Here's how the part is built. I have some questions about the finished solid (model axes, mm). A direction names the side the tool comes from. Round coordinates to 2 decimals unless told otherwise and drop trailing zeros. Write each loop counter-clockwise with the first axis right and the second up, starting at its lowest first coordinate (ties: lowest second). Pieces come first, ordered by that corner, then holes. Notation, with made-up numbers: (48, -1.5) -> (105, -1.5) arc R8 cw to (105, 7.5) -> close; hole circle Ø7 at (-5, -38.5). An arc over 180 degrees is marked (long way). Answer as CSV lines item,"result".
from build123d import *

# Parameters (mm, degrees)
SKETCH1_R           = 11
BOSS_EXTRUDE2_DEPTH = 13
SKETCH4_W           = 38
SKETCH4_H           = 51
BOSS_EXTRUDE3_DEPTH = 45
CUT_EXTRUDE1_DEPTH  = 45
BOSS_EXTRUDE4_DEPTH = 45
SKETCH15_R          = 11
BOSS_EXTRUDE6_DEPTH = 10
SKETCH16_R          = 11
BOSS_EXTRUDE7_DEPTH = 10


with BuildPart() as part:
    # Sketch1 → Boss-Extrude2 (new body)
    with BuildSketch(Plane(origin=(0, 0, 0), x_dir=(1, 0, 0), z_dir=(0, 1, 0))):
        with BuildLine():
            Line((-57, 32), (57, 32))
            ThreePointArc((57, 32), (89, 0), (57, -32))
            Line((57, -32), (-57, -32))
            ThreePointArc((-57, -32), (-89, 0), (-57, 32))
        make_face()
        with Locations(Location((-57, 0, 0), (0, 0, 90))):
            Circle(SKETCH1_R, mode=Mode.SUBTRACT)
        with Locations(Location((57, 0, 0), (0, 0, 90))):
            Circle(SKETCH1_R, mode=Mode.SUBTRACT)
    extrude(amount=BOSS_EXTRUDE2_DEPTH)

    # Sketch4 → Boss-Extrude3 (add)
    with BuildSketch(Plane(origin=(0, 13, 0), x_dir=(1, 0, 0), z_dir=(0, 1, 0))):
        with Locations((0, -6.5)):
            Rectangle(SKETCH4_W, SKETCH4_H)
    extrude(amount=BOSS_EXTRUDE3_DEPTH)

    # Sketch5 → Cut-Extrude1 (cut)
    with BuildSketch(Plane(origin=(19, 0, 0), x_dir=(0, 0, -1), z_dir=(1, 0, 0))):
        Polygon((19, 58), (-32, 13), (-32, 58), align=None)
    extrude(amount=-CUT_EXTRUDE1_DEPTH, mode=Mode.SUBTRACT)

    # Sketch6 → Boss-Extrude4 (add)
    with BuildSketch(Plane(origin=(0, 13, 0), x_dir=(1, 0, 0), z_dir=(0, 1, 0))):
        Polygon((-32, 32), (-32, -32), (-19, -32), (-19, 19), (19, 19), (19, -32), (32, -32), (32, 32), align=None)
    extrude(amount=BOSS_EXTRUDE4_DEPTH)

    # Sketch15 → Boss-Extrude6 (add)
    with BuildSketch(Plane(origin=(0, 13, 0), x_dir=(1, 0, 0), z_dir=(0, 1, 0))):
        with BuildLine():
            Line((-32, 32), (-57, 32))
            ThreePointArc((-57, 32), (-89, 0), (-57, -32))
            Line((-57, -32), (-32, -32))
            Line((-32, -32), (-32, 32))
        make_face()
        with Locations(Location((-57, 0, 0), (0, 0, 90))):
            Circle(SKETCH15_R, mode=Mode.SUBTRACT)
    extrude(amount=BOSS_EXTRUDE6_DEPTH)

    # Sketch16 → Boss-Extrude7 (add)
    with BuildSketch(Plane(origin=(0, 13, 0), x_dir=(1, 0, 0), z_dir=(0, 1, 0))):
        with BuildLine():
            Line((32, -32), (57, -32))
            ThreePointArc((57, -32), (89, 0), (57, 32))
            Line((57, 32), (32, 32))
            Line((32, 32), (32, -32))
        make_face()
        with Locations(Location((57, 0, 0), (0, 0, 90))):
            Circle(SKETCH16_R, mode=Mode.SUBTRACT)
    extrude(amount=BOSS_EXTRUDE7_DEPTH)


solid = part.part
Item 1: Will these pins go through, and if not, where does the flat tip stop? pin 1 (6 mm diameter, centred on x = 6.5, z = 23.5, fed in from +Y); pin 2 (8 mm diameter, centred on x = -46.5, z = -21, fed in from +Y); pin 3 (22.5 mm diameter, centred on y = 42, z = 14.5, fed in from -X).
Results found:
pin 1,"stops at y = 23.15"
pin 2,"stops at y = 23"
pin 3,"stops at x = -32"
Item 2: If we mould it in two halves opening along Z, with no side actions, what happens to faces 6 (the flat face through (1, 0, 0)), 7 (the cylindrical face through (46.094, 11.339, 1.432)), 8 (the cylindrical face through (-88.992, 11.339, -0.704)), 9 (the cylindrical face through (-67.906, 11.339, 1.432))? For each: pulls with the +Z half, pulls with the -Z half, needs draft (parallel to the pull), parting line crosses it, or undercut.
Results found:
face 6,"needs draft"
face 7,"undercut"
face 8,"parting line crosses it"
face 9,"undercut"
Item 3: For faces 1 (the flat face through (66, 23, -8)), 2 (the flat face through (-32, 40, 0)), 3 (the flat face through (0, 58, -22)), 4 (the flat face through (-19, 45, 18)), 5 (the cylindrical face through (88.992, 11.339, 0.704)), which set-ups out of +Z, -Z, +X, -X, +Y, -Y let a thin tool reach every point of the face, with its end or its side?
Results found:
face 1,"+Z, -Z, +X, +Y"
face 2,"+Z, -Z, -X, +Y"
face 3,"+Z, -Z, +X, -X, +Y"
face 4,"+Z, +Y"
face 5,"+X, +Y, -Y"
Item 4: Suppose I cut it at D-D, the plane x = 6. List the corners of the cut face in (y, z) for me.
Results found:
outline,"(0, -32) -> (58, -32) -> (58, -19) -> (13, 32) -> (0, 32) -> close"
Item 5: I need wall thicknesses on L1, parallel to X at y = 11.75, z = 0; L2, parallel to Z at x = -57, y = 6; L3, parallel to X at y = 14, z = -8. Which ranges of each line are inside material? Lowest first, please.
Results found:
L1,"x = -89 to -68, -46 to 46, 68 to 89"
L2,"z = -32 to -11, 11 to 32"
L3,"x = -87.98 to -64.55, -49.45 to 49.45, 64.55 to 87.98"
Item 6: Suppose I cut it at C-C, the plane y = 52. List the corners of the cut face in (x, z) for me.
Results found:
outline,"(-32, -32) -> (32, -32) -> (32, 32) -> (19, 32) -> (19, -12.2) -> (-19, -12.2) -> (-19, 32) -> (-32, 32) -> close"
Item 7: Suppose I cut it at A-A, the plane z = 0. List the corners of the cut face in (x, y) for me, then the cut area to 3 significant figures.
Results found:
outline,"(-89, 0) -> (-68, 0) -> (-68, 23) -> (-89, 23) -> close; (-46, 0) -> (46, 0) -> (46, 23) -> (32, 23) -> (32, 58) -> (19, 58) -> (19, 41.24) -> (-19, 41.24) -> (-19, 58) -> (-32, 58) -> (-32, 23) -> (-46, 23) -> close; (68, 0) -> (89, 0) -> (89, 23) -> (68, 23) -> close"
area,"4,680 mm²"
Item 8: Suppose I cut it at B-B, the plane y = 21. List the corners of the cut face in (x, z) for me, then the cut area to 3 significant figures.
Results found:
outline,"(-57, -32) -> (57, -32) arc R32 ccw to (57, 32) -> (19, 32) -> (19, 22.93) -> (-19, 22.93) -> (-19, 32) -> (-57, 32) arc R32 ccw to start; hole circle Ø22 at (-57, 0); hole circle Ø22 at (57, 0)"
area,"9,410 mm²"
